The model under review builds one solid part; all positions refer to its coordinate system, in mm. A direction names the side the tool comes from. Give positions to 0.01 mm unless a question says otherwise; leave off trailing zeros. Write each loop counter-clockwise with the first axis right and the second up, starting at its lowest first coordinate (ties: lowest second). Pieces come first, ordered by that corner, then holes. Notation, with made-up numbers: M 21.25,46 L 47.25,46 A26 ccw 47.25,83 Z; hole C 3,24.25 d5. An arc over 180 degrees is marked long. Write item = value, one per line. Start each with the question number.
```python
from build123d import *

# Parameters (mm, degrees)
ESQUISSE1_W             = 40
ESQUISSE1_H             = 32
EXTRUSION1_DEPTH        = 10
ESQUISSE2_R             = 6.5
EXTRUSION2_DEPTH        = 1
CONG_1_R                = 0.8
ESQUISSE3_R             = 3
EXTRUSION3_DEPTH        = 4.5
ESQUISSE4_W             = 9
ESQUISSE4_H             = 7
EXTRUSION4_DEPTH        = 3.5
EXTRUSION4_DEPTH_BACK   = 1
ESQUISSE5_W             = 1.3
ESQUISSE5_H             = 1.1
ENL_V_MAT_EXTRU_2_DEPTH = 3.5
ENL_V_MAT_EXTRU_5_REACH = 14.4
ESQUISSE9_W             = 1.3
ESQUISSE9_H             = 1.1
ESQUISSE7_R             = 1
ENL_V_MAT_EXTRU_4_DEPTH = 4.5
ESQUISSE8_W             = 7.5
ESQUISSE8_H             = 2.6
EXTRUSION6_DEPTH        = 20
EXTRUSION7_DEPTH        = 1
ENL_V_MAT_EXTRU_6_REACH = 29.1
ESQUISSE11_R            = 2.5


with BuildPart() as part:
    # Esquisse1 → Extrusion1 (new body, symmetric)
    with BuildSketch(Plane.XY):
        with Locations((20, 16)):
            Rectangle(ESQUISSE1_W, ESQUISSE1_H)
    extrude(amount=EXTRUSION1_DEPTH, both=True)

    # Esquisse2 → Extrusion2 (add)
    with BuildSketch(Plane(origin=(0, 32, 0), x_dir=(-1, 0, 0), z_dir=(0, 1, 0))):
        with Locations((-30, 0)):
            Circle(ESQUISSE2_R)
    extrude(amount=EXTRUSION2_DEPTH)

    # Cong_1
    cong_1_edges = [part.edges().sort_by_distance(p)[0] for p in [
        (36.5, 33, 0),
    ]]
    fillet(cong_1_edges, radius=CONG_1_R)

    # Esquisse3 → Extrusion3 (add)
    with BuildSketch(Plane(origin=(0, 33, 0), x_dir=(-1, 0, 0), z_dir=(0, 1, 0))):
        with Locations((-30, 0)):
            Circle(ESQUISSE3_R)
    extrude(amount=EXTRUSION3_DEPTH)

    # Esquisse4 → Extrusion4 (add, two sides)
    with BuildSketch(Plane.XZ) as extrusion4_sk:
        with Locations((42, 0)):
            Rectangle(ESQUISSE4_W, ESQUISSE4_H)
    extrude(amount=EXTRUSION4_DEPTH)
    extrude(extrusion4_sk.sketch, amount=-EXTRUSION4_DEPTH_BACK)

    # Esquisse5 → Enl_v. mat.-Extru.2 (cut)
    with BuildSketch(Plane.XZ.offset(3.5)):
        with Locations((39.35, 2.95)):
            Rectangle(ESQUISSE5_W, ESQUISSE5_H)
        with Locations((39.35, -2.95)):
            Rectangle(ESQUISSE5_W, ESQUISSE5_H)
    extrude(amount=-ENL_V_MAT_EXTRU_2_DEPTH, mode=Mode.SUBTRACT)

    # Esquisse9 → Enl_v. mat.-Extru.5 (cut, up to next)
    with BuildSketch(Plane(origin=(0, 0, -2.4), x_dir=(-1, 0, 0), z_dir=(0, 0, -1)), mode=Mode.PRIVATE) as enl_v_mat_extru_5_sk1:
        with Locations((-39.35, -2.95)):
            Rectangle(ESQUISSE9_W, ESQUISSE9_H)
    enl_v_mat_extru_5_tool1 = extrude(enl_v_mat_extru_5_sk1.sketch, amount=-ENL_V_MAT_EXTRU_5_REACH, mode=Mode.PRIVATE) & part.part
    add(enl_v_mat_extru_5_tool1.solids().sort_by_distance((39.35, -2.95, -2.4))[0], mode=Mode.SUBTRACT)

    # Esquisse7 → Enl_v. mat.-Extru.4 (cut)
    with BuildSketch(Plane.XZ):
        with Locations((37.3, -7.3)):
            Circle(ESQUISSE7_R)
        with Locations((2.7, -7.3)):
            Circle(ESQUISSE7_R)
        with Locations((2.7, 7.3)):
            Circle(ESQUISSE7_R)
        with Locations((37.3, 7.3)):
            Circle(ESQUISSE7_R)
    extrude(amount=-ENL_V_MAT_EXTRU_4_DEPTH, mode=Mode.SUBTRACT)

    # Esquisse8 → Extrusion6 (add)
    with BuildSketch(Plane.XY.offset(10)):
        with Locations((43.75, 22.3)):
            Rectangle(ESQUISSE8_W, ESQUISSE8_H)
        with Locations((-3.75, 22.3)):
            Rectangle(ESQUISSE8_W, ESQUISSE8_H)
    extrude(amount=-EXTRUSION6_DEPTH)

    # Esquisse10 → Extrusion7 (add, symmetric)
    with BuildSketch(Plane.XY):
        Polygon((40, 26.6), (40, 23.6), (44.8, 23.6), align=None)
        Polygon((-4.8, 23.6), (0, 23.6), (0, 26.6), align=None)
    extrude(amount=EXTRUSION7_DEPTH, both=True)

    # Esquisse11 → Enl_v. mat.-Extru.6 (cut, up to next)
    with BuildSketch(Plane(origin=(0, 23.6, 0), x_dir=(-1, 0, 0), z_dir=(0, 1, 0)), mode=Mode.PRIVATE) as enl_v_mat_extru_6_sk1:
        with Locations((-44.5, 5)):
            Circle(ESQUISSE11_R)
    enl_v_mat_extru_6_tool1 = extrude(enl_v_mat_extru_6_sk1.sketch, amount=-ENL_V_MAT_EXTRU_6_REACH, mode=Mode.PRIVATE) & part.part
    add(enl_v_mat_extru_6_tool1.solids().sort_by_distance((44.5, 23.6, 5))[0], mode=Mode.SUBTRACT)
    # Esquisse11 → Enl_v. mat.-Extru.6 (cut, up to next)
    with BuildSketch(Plane(origin=(0, 23.6, 0), x_dir=(-1, 0, 0), z_dir=(0, 1, 0)), mode=Mode.PRIVATE) as enl_v_mat_extru_6_sk2:
        with Locations((-44.5, -5)):
            Circle(ESQUISSE11_R)
    enl_v_mat_extru_6_tool2 = extrude(enl_v_mat_extru_6_sk2.sketch, amount=-ENL_V_MAT_EXTRU_6_REACH, mode=Mode.PRIVATE) & part.part
    add(enl_v_mat_extru_6_tool2.solids().sort_by_distance((44.5, 23.6, -5))[0], mode=Mode.SUBTRACT)
    # Esquisse11 → Enl_v. mat.-Extru.6 (cut, up to next)
    with BuildSketch(Plane(origin=(0, 23.6, 0), x_dir=(-1, 0, 0), z_dir=(0, 1, 0)), mode=Mode.PRIVATE) as enl_v_mat_extru_6_sk3:
        with Locations((4.5, -5)):
            Circle(ESQUISSE11_R)
    enl_v_mat_extru_6_tool3 = extrude(enl_v_mat_extru_6_sk3.sketch, amount=-ENL_V_MAT_EXTRU_6_REACH, mode=Mode.PRIVATE) & part.part
    add(enl_v_mat_extru_6_tool3.solids().sort_by_distance((-4.5, 23.6, -5))[0], mode=Mode.SUBTRACT)
    # Esquisse11 → Enl_v. mat.-Extru.6 (cut, up to next)
    with BuildSketch(Plane(origin=(0, 23.6, 0), x_dir=(-1, 0, 0), z_dir=(0, 1, 0)), mode=Mode.PRIVATE) as enl_v_mat_extru_6_sk4:
        with Locations((4.5, 5)):
            Circle(ESQUISSE11_R)
    enl_v_mat_extru_6_tool4 = extrude(enl_v_mat_extru_6_sk4.sketch, amount=-ENL_V_MAT_EXTRU_6_REACH, mode=Mode.PRIVATE) & part.part
    add(enl_v_mat_extru_6_tool4.solids().sort_by_distance((-4.5, 23.6, 5))[0], mode=Mode.SUBTRACT)


solid = part.part
```
Item 1: Clearance check with flat-ended pins moving along their axes: P1, Ø1.4, axis at x = 39.5, y = -1, coming from the -Z side; P2, Ø4, axis at y = 30, z = 5, coming from the +X side; P3, Ø1.5, axis at x = -1.5, y = 25.5, coming from the +Z side. State where each tip first meets the part, or that it passes through.
Item 2: For faces 4 (the flat face through (40, -3, 0)), 5 (the flat face through (39, -2.4, 0)), 6 (the flat face through (41, 24, -1)), 7 (the flat face through (0, 28, 0)), list the 3-axis set-ups (+Z, -Z, +X, -X, +Y, -Y) from which the entire face can be reached by the end or side of a thin tool; tool diameter is ignored.
Item 3: We need section D-D, the plane y = 10.5. Write out the cut boundary in (x, z), and give its area (3 significant figures).
Item 4: We need section B-B, the plane y = 24.5. Write out the cut boundary in (x, z), and give its area (3 significant figures).
Item 5: We need section C-C, the plane x = 8. Write out the cut boundary in (y, z), and give its area (3 significant figures).
Item 6: To check wall thickness, follow probe 1 along Z at (x, y) = (44.5, 21.85); probe 2 along Z at (x, y) = (2.7, 1.65); probe 3 along X at (y, z) = (17.5, -4.5). State the ranges of each line that lie inside material, in increasing order. Write a range as [from, to].
Item 7: The part is to be moulded in two halves that separate along Z. For faces 1 (the flat face through (-4, 21, 0)), 2 (the cylindrical face through (1.963, 2.218, 7.976)), 3 (the flat face through (39, -1, -2.4)), say which applies: released by +Z, released by -Z, zero draft, split by the parting line, or undercut.
Worked out:
q1.P1 = -3.5
q1.P2 = 40
q1.P3 = 1
q2.face_4 = -Y
q2.face_5 = +Z, -Z, -Y
q2.face_6 = -Z, +X, +Y
q2.face_7 = -X, +Y
q3.outline = M 0,-10 L 40,-10 L 40,10 L 0,10 Z
q3.area = 800 mm²
q4.outline = M -3.36,-1 L 0,-1 L 0,-10 L 40,-10 L 40,-1 L 43.36,-1 L 43.36,1 L 40,1 L 40,10 L 0,10 L 0,1 L -3.36,1 Z
q4.area = 813 mm²
q5.outline = M 0,-10 L 32,-10 L 32,10 L 0,10 Z
q5.area = 640 mm²
q6.probe_1 = [-10, -7.5], [-2.5, 2.5], [7.5, 10]
q6.probe_2 = [-10, -8.3], [-6.3, 6.3], [8.3, 10]
q6.probe_3 = [0, 40]
q7.face_1 = zero draft
q7.face_2 = undercut
q7.face_3 = released by -Z
